Verification items for this drawing (mm, ordinates from the low corner). A direction names the side the tool comes from. Round coordinates to 2 decimals unless told otherwise and drop trailing zeros. Loops run counter-clockwise (first coordinate to the right, second up) from the corner with the lowest first, then second, coordinate; pieces in that order, holes last. Notation, with made-up numbers: M 52,-36.75 L 103,-36.75 A8 cw 103,-24.75 Z; hole C 38,36 d8. An arc over 180 degrees is marked long. Write item = value, one per line.
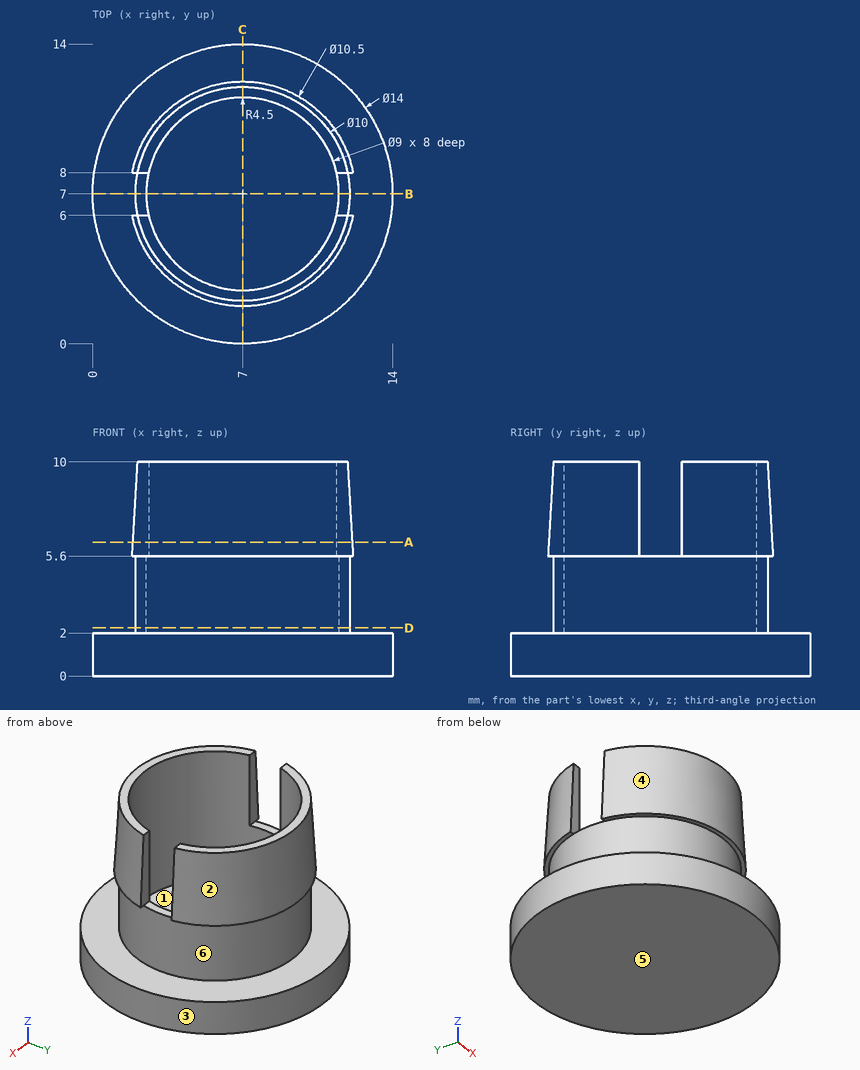
(1) Sectioned sample at D-D on z = 2.25. Record the cut outline in (x, y), then the cut area to 3 significant figures.
Result set:
outline = C 7,7 d10; hole C 7,7 d9
area = 14.9 mm2
(2) Release check for a two-part mould opening along Z. For the marked faces 3, 4, 5 and 6 record: released by +Z, released by -Z, zero draft, split by the parting line, or undercut.
Result set:
face_3 = zero draft
face_4 = released by +Z
face_5 = released by -Z
face_6 = undercut
(3) Sectioned sample at A-A on z = 6.25. Record the cut outline in (x, y), then the cut area to 3 significant figures.
Result set:
outline = M 1.88,6 A5.21 ccw 12.12,6 L 11.39,6 A4.5 cw 2.61,6 Z; M 1.88,8 L 2.61,8 A4.5 cw 11.39,8 L 12.12,8 A5.21 ccw Z
area = 18.9 mm2
(4) Material ranges on line 1 along Z through (x, y) = (3.25, 1.75); line 2 along X through (y, z) = (7.25, 4); line 3 along X through (y, z) = (9.75, 4.75), recorded low to high. Write a range as from..to.
Result set:
line_1 = 0..2
line_2 = 2.01..2.51, 11.49..11.99
line_3 = 2.82..3.44, 10.56..11.18
(5) Sectioned sample at B-B on y = 7. Record the cut outline in (x, z), then the cut area to 3 significant figures.
Result set:
outline = M 0,0 L 14,0 L 14,2 L 12,2 L 12,5.6 L 11.5,5.6 L 11.5,2 L 2.5,2 L 2.5,5.6 L 2,5.6 L 2,2 L 0,2 Z
area = 31.6 mm2
(6) Depth check by flat-ended pin: pin 1 Ø1.5 at (x, z) = (9, 7.5) entering from -Y; pin 2 Ø7 at (x, y) = (7, 7) entering from -Z; pin 3 Ø0.7 at (x, y) = (11.5, 7.5) entering from +Z; pin 4 Ø3 at (x, z) = (2, 8.5) entering from +Y. Enter the tip coordinate at first touch or a pass-through.
Result set:
pin_1 = 2.01
pin_2 = 0
pin_3 = 5.6
pin_4 = 10.69
(7) Tool access check on the marked faces 1 and 2. Record the directions out of +Z, -Z, +X, -X, +Y, -Y that give a thin tool (end or side, any length) a straight path to the whole face; none if there is none.
Result set:
face_1 = +Z
face_2 = +Z, +Y
(8) Sectioned sample at C-C on x = 7. Record the cut outline in (y, z).
Result set:
outline = M 0,0 L 14,0 L 14,2 L 12,2 L 12,5.6 L 12.25,5.6 L 12,10 L 11.5,10 L 11.5,2 L 2.5,2 L 2.5,10 L 2,10 L 1.75,5.6 L 2,5.6 L 2,2 L 0,2 Z
